```python
from build123d import *

# Parameters (mm, degrees)
EXTRUDE_1_DEPTH        = 54
EXTRUDE_2_DEPTH        = 10
SKETCH_3_W             = 6.5
SKETCH_3_H             = 20
CUT_EXTRUDE_1_DEPTH    = 10
EXTRUDE_3_DEPTH        = 15
EXTRUDE_4_DEPTH        = 15
PATTERN_LINEAR_6_COUNT = 2
PATTERN_LINEAR_6_PITCH = 18
SKETCH_8_W             = 3
SKETCH_8_H             = 3
CUT_EXTRUDE_2_DEPTH    = 73.562318045
SKETCH_9_R             = 2.5
EXTRUDE_5_DEPTH        = 8
OTHER_START            = -10
OTHER_1_OUTLINE_R      = 2.3
OTHER_1_DEPTH          = 20
OTHER_1_2_OUTLINE_R    = 3.6
OTHER_1_2_OUTLINE_R_2  = 2.3
OTHER_1_2_DEPTH        = 1


# Read off the part's stored shape, not the designer's step: 高级异型孔1, 高级异型孔2
with BuildPart() as part:
    # 草图1 → 凸台-拉伸1 (new body)
    with BuildSketch(Plane(origin=(0, 0, 0), x_dir=(1, 0, 0), z_dir=(0, 1, 0))):
        Polygon((-12.038834765, 10), (-16.35, 10), (-16.35, -10), (16.35, -10), (16.35, 10), (12.038834765, 10), (0, -2.038834765), align=None)
    extrude(amount=EXTRUDE_1_DEPTH)

    # 草图2 → 凸台-拉伸2 (add)
    with BuildSketch(Plane(origin=(0, 54, 0), x_dir=(1, 0, 0), z_dir=(0, 1, 0))):
        Polygon((16.35, 10), (12.038834765, 10), (0, -2.038834765), (-12.038834765, 10), (-16.35, 10), (-16.35, -10), (16.35, -10), align=None)
        Polygon((12.038834765, 10), (-12.038834765, 10), (0, -2.038834765), align=None)
    extrude(amount=EXTRUDE_2_DEPTH)

    # 草图3 → 切除-拉伸1 (cut)
    with BuildSketch(Plane(origin=(0, 64, 0), x_dir=(1, 0, 0), z_dir=(0, 1, 0))):
        Rectangle(SKETCH_3_W, SKETCH_3_H)
    extrude(amount=-CUT_EXTRUDE_1_DEPTH, mode=Mode.SUBTRACT)

    # 草图5 → 凸台-拉伸3 (add)
    with BuildSketch(Plane(origin=(0, 0, 0), x_dir=(-1, 0, 0), z_dir=(0, -1, 0))):
        Polygon((6.25, 4.211165235), (12.038834765, 10), (6.25, 10), align=None)
        Polygon((-6.25, 4.211165235), (-12.038834765, 10), (-6.25, 10), align=None)
    extrude(amount=-EXTRUDE_3_DEPTH)

    # 草图6 → 凸台-拉伸4 (add)
    with BuildSketch(Plane(origin=(0, 18, 0), x_dir=(1, 0, 0), z_dir=(0, 1, 0))):
        Polygon((12.038834765, 10), (6.25, 10), (6.25, 4.211165235), align=None)
        Polygon((-6.25, 4.211165235), (-12.038834765, 10), (-6.25, 10), align=None)
    extrude_4 = extrude(amount=EXTRUDE_4_DEPTH)

    # 阵列(线性)6: 凸台-拉伸4 ×2
    with Locations(*[(0, i * PATTERN_LINEAR_6_PITCH, 0) for i in range(1, PATTERN_LINEAR_6_COUNT)]):
        add(extrude_4)

    # 草图8 → 切除-拉伸2 (cut, through all)
    with BuildSketch(Plane(origin=(16.35, 0, 0), x_dir=(0, 0, -1), z_dir=(1, 0, 0))):
        with Locations((8.5, 52.5)):
            Rectangle(SKETCH_8_W, SKETCH_8_H)
        with Locations((8.5, 34.5)):
            Rectangle(SKETCH_8_W, SKETCH_8_H)
        with Locations((8.5, 16.5)):
            Rectangle(SKETCH_8_W, SKETCH_8_H)
    extrude(amount=-CUT_EXTRUDE_2_DEPTH, mode=Mode.SUBTRACT)

    # 草图9 → 凸台-拉伸5 (add)
    with BuildSketch(Plane(origin=(0, 0, -10), x_dir=(-1, 0, 0), z_dir=(0, 0, -1))):
        with Locations((-11.3, 43.5)):
            Circle(SKETCH_9_R)
        with Locations((11.3, 43.5)):
            Circle(SKETCH_9_R)
        with Locations(Location((11.3, 7.5, 0), (0, 0, 180))):
            Circle(SKETCH_9_R)
        with Locations(Location((-11.3, 7.5, 0), (0, 0, 180))):
            Circle(SKETCH_9_R)
    extrude(amount=EXTRUDE_5_DEPTH)

    # 高级异型孔1 outline → 高级异型孔1 (cut)
    with BuildSketch(Plane.XY.offset(OTHER_START)):
        with Locations((-11.3, 25.5)):
            Circle(OTHER_1_OUTLINE_R)
        with Locations((11.3, 25.5)):
            Circle(OTHER_1_OUTLINE_R)
    extrude(amount=OTHER_1_DEPTH, mode=Mode.SUBTRACT)

    # Other 1 2 outline → Other 1 2 (cut)
    # profile 1 of 2: a face of its own
    with BuildSketch(Plane.XY.offset(OTHER_START)):
        with Locations((-11.3, 25.5)):
            Circle(OTHER_1_2_OUTLINE_R)
        with Locations((-11.3, 25.5)):
            Circle(OTHER_1_2_OUTLINE_R_2, mode=Mode.SUBTRACT)
    # profile 2 of 2: a face of its own
    with BuildSketch(Plane.XY.offset(OTHER_START)):
        with Locations((11.3, 25.5)):
            Circle(OTHER_1_2_OUTLINE_R)
        with Locations((11.3, 25.5)):
            Circle(OTHER_1_2_OUTLINE_R_2, mode=Mode.SUBTRACT)
    extrude(amount=OTHER_1_2_DEPTH, mode=Mode.SUBTRACT)

    # 高级异型孔2 outline → 高级异型孔2 (revolve, cut)
    with BuildSketch(Plane(origin=(0, 34.5, 4.998489893), x_dir=(0, 1, 0), z_dir=(0, 0, -1))):
        Polygon((3.6, -16.35), (3.6, -15.35), (2.3, -15.35), (2.3, -5.35), (0, -3.96802058), (0, -16.35), align=None)
    other_2 = revolve(axis=Axis((0, 34.5, 4.998489893), (1, 0, 0)), mode=Mode.SUBTRACT)

    # Other 2 2 outline → Other 2 2 (revolve, cut)
    with BuildSketch(Plane(origin=(0, 16.5, 4.998489893), x_dir=(0, 1, 0), z_dir=(0, 0, -1))):
        Polygon((0, -16.35), (3.6, -16.35), (3.6, -15.35), (2.3, -15.35), (2.3, -5.35), (0, -3.96802058), align=None)
    other_2_2 = revolve(axis=Axis((0, 16.5, 4.998489893), (1, 0, 0)), mode=Mode.SUBTRACT)

    # 镜向1: 高级异型孔2, Other 2 2 across plane
    add(other_2.mirror(Plane(origin=(0, 0, 0), x_dir=(0, 0, 1), z_dir=(1, 0, 0))), mode=Mode.SUBTRACT)
    add(other_2_2.mirror(Plane(origin=(0, 0, 0), x_dir=(0, 0, 1), z_dir=(1, 0, 0))), mode=Mode.SUBTRACT)


solid = part.part
```
Could you check a few things on this model? Use its own coordinates, in mm. A direction names the side the tool comes from. Coordinates: 2 decimals unless noted, no trailing zeros. Loops run counter-clockwise (first coordinate to the right, second up) from the corner with the lowest first, then second, coordinate; pieces in that order, holes last. Notation, with made-up numbers: M 47,65.25 L 85,65.25 A15 cw 85,93.25 Z; hole C 74.25,19 d10. An arc over 180 degrees is marked long. Put each result on its own line as item: value. Start each with the question number.
(1) Will these pins go through, and if not, where does the flat tip stop? P1, Ø5, axis at x = -10, y = 22, coming from the -Z side; P2, Ø6, axis at x = 11.3, y = 25.5, coming from the -Z side; P3, Ø4, axis at y = 46, z = -13.5, coming from the +X side.
(2) Suppose I cut it at B-B on x = -11.3. Count the separate pieces of the cut face and the enclosed holes in it, then the cut area to 3 significant figures.
(3) Suppose I cut it at A-A on y = 25.5. Please give me the cut outline in (x, z), then the cut area to 3 significant figures.
(4) Thinking about a two-plate mould opening in Z: for faces 4 (the face through (14, 42, -10)), 5 (the face through (-11, 36, -8)), 6 (the face through (-15.843, 13.847, 7.432)), which applies, pulls with the +Z half, pulls with the -Z half, needs draft (parallel to the pull), parting line crosses it, or undercut?
(5) I need wall thicknesses on line 1 (Y direction, x = 8.5, z = -7.75); line 2 (Z direction, x = 16, y = 34.5); line 3 (X direction, y = 49, z = -4.5). Which ranges of each line are inside material? Lowest first, please. Write a range as from..to.
(6) For faces 1 (the face through (-3.25, 59, 0)), 2 (the face through (11.84, 41.06, -13.94)), 3 (the face through (-15, 24, -10)), which set-ups out of +Z, -Z, +X, -X, +Y, -Y let a thin tool reach every point of the face, with its end or its side?
(7) Suppose I cut it at D-D on y = 7.5. Please give me the cut outline in (x, z), then the cut area to 3 significant figures.
Solutions:
1. P1: stops at z = -10
1. P2: stops at z = -9
1. P3: stops at x = 13.75
2. separate pieces: 2
2. enclosed holes: 2
2. area: 1,210 mm2
3. outline: M -16.35,-10 L -14.9,-10 L -14.9,-9 L -13.6,-9 L -13.6,10 L -16.35,10 Z; M -9,-9 L -7.7,-9 L -7.7,-10 L -6.25,-10 L -6.25,-4.21 L 0,2.04 L 6.25,-4.21 L 6.25,-10 L 7.7,-10 L 7.7,-9 L 9,-9 L 9,10 L -9,10 Z; M 13.6,-9 L 14.9,-9 L 14.9,-10 L 16.35,-10 L 16.35,10 L 13.6,10 Z
3. area: 353 mm2
4. face 4: pulls with the -Z half
4. face 5: needs draft
4. face 6: undercut
5. line 1: y = 0..15, 18..33, 36..51, 54..64
5. line 2: z = -7..1.4, 8.6..10
5. line 3: x = -16.35..-6.25, 6.25..16.35
6. face 1: +Z, -Z, +Y
6. face 2: -Z
6. face 3: -Z, +X, -X
7. outline: M -16.35,-10 L -13.8,-10 L -13.8,-18 L -8.8,-18 L -8.8,-10 L -6.25,-10 L -6.25,-4.21 L 0,2.04 L 6.25,-4.21 L 6.25,-10 L 8.8,-10 L 8.8,-18 L 13.8,-18 L 13.8,-10 L 16.35,-10 L 16.35,10 L -16.35,10 Z
7. area: 623 mm2
